Read the model definition and answer for the solid it produces. Units are mm, in the model's axes. A direction names the side the tool comes from. Coordinates: 2 decimals unless noted, no trailing zeros. Write each loop counter-clockwise with the first axis right and the second up, starting at its lowest first coordinate (ties: lowest second). Pieces come first, ordered by that corner, then holes.
Item 1: Determine the mould class of faces 1 (the face through (-4, 10, -17)), 2 (the face through (227, 15, -17)), 3 (the face through (-14, 0, -12)), 4 (the face through (232.3, 0, -11)) for opening direction X: released by +X, released by -X, zero draft, split by the parting line, or undercut.
Item 2: Straight lines are drawn through the part: probe 1 along X at (y, z) = (2, -13); probe 2 along Z at (x, y) = (94, -0.5); probe 3 along X at (y, z) = (6, -16). For each, find the intervals that lie inside material, in ascending order.
Item 3: Section A-A (y = -9) is taken. Give the vertices of the cut face in (x, z), then the cut area to 3 significant figures.
Item 4: Section D-D (x = 36) is taken. Give the vertices of the cut face in (y, z), then the cut area to 3 significant figures.
Item 5: A tool of negligible diameter and unlimited length cuts with its end or side. For faces 5 (the face through (222.3, 10, -17)), 6 (the face through (108, -5, -17)), 7 (the face through (-12, 5.63, -7)), 8 (the face through (228.3, 0, -7)), from which of +Z, -Z, +X, -X, +Y, -Y can it reach the whole face along a straight path? Write none if from no direction.
Item 6: Section B-B (z = -5.5) is taken. Give the vertices of the cut face in (x, y), then the cut area to 3 significant figures.
Item 7: Section C-C (y = 0) is taken. Give the vertices of the cut face in (x, z).
Item 8: Each of these flat-tipped pins is pushed along its axis until it touches: P1, Ø4.5, axis at x = 230, z = -7.5, coming from the -Y side; P2, Ø4.5, axis at x = 99.5, z = -17, coming from the -Y side; P3, Ø2, axis at x = 229.5, z = -10.5, coming from the +Y side. Where does it stop, or does it pass through?
from build123d import *

# Parameters (mm, degrees)
EXTRUDE_START   = -15
SKETCH_1_W      = 246.3
SKETCH_1_H      = 10
EXTRUDE_1_DEPTH = 4
SKETCH_2_W      = 10
SKETCH_2_H      = 30
EXTRUDE_2_DEPTH = 4
EXTRUDE_3_DEPTH = 4
EXTRUDE_START_2 = -4
EXTRUDE_4_DEPTH = 4


with BuildPart() as part:
    # 草图1 → 凸台-拉伸1 (new body)
    with BuildSketch(Plane.XY.offset(EXTRUDE_START)):
        with Locations((109.15, 0)):
            Rectangle(SKETCH_1_W, SKETCH_1_H)
    extrude(amount=-EXTRUDE_1_DEPTH)

    # 草图2 → 凸台-拉伸2 (add)
    with BuildSketch(Plane(origin=(0, 0, -19), x_dir=(-1, 0, 0), z_dir=(0, 0, -1))):
        with Locations((9, 0)):
            Rectangle(SKETCH_2_W, SKETCH_2_H)
        with Locations((-227.3, 0)):
            Rectangle(SKETCH_2_W, SKETCH_2_H)
    extrude(amount=-EXTRUDE_2_DEPTH)

    # 草图4 → 凸台-拉伸3 (add)
    with BuildSketch(Plane(origin=(232.3, 0, 0), x_dir=(0, 0, -1), z_dir=(1, 0, 0))):
        with BuildLine():
            Line((0, -2.63), (0, -5.63))
            Line((0, -5.63), (15, -5.63))
            Line((15, -5.63), (15, 5.63))
            Line((15, 5.63), (0, 5.63))
            Line((0, 5.63), (0, 2.63))
            ThreePointArc((0, 2.63), (2.63, 0), (0, -2.63))
        make_face()
    extrude(amount=-EXTRUDE_3_DEPTH)

    # 草图5 → 凸台-拉伸4 (add)
    with BuildSketch(Plane.ZY.offset(14).offset(EXTRUDE_START_2)):
        with BuildLine():
            Line((0, 2.63), (0, 5.63))
            Line((0, 5.63), (-15, 5.63))
            Line((-15, 5.63), (-15, -5.63))
            Line((-15, -5.63), (0, -5.63))
            Line((0, -5.63), (0, -2.63))
            ThreePointArc((0, -2.63), (-2.63, 0), (0, 2.63))
        make_face()
    extrude(amount=EXTRUDE_4_DEPTH)


solid = part.part
Established:
1. face 1: undercut
1. face 2: zero draft
1. face 3: released by -X
1. face 4: released by +X
2. probe 1: x = -14 to -10, 228.3 to 232.3
2. probe 2: z = -19 to -15
2. probe 3: x = -14 to -4, 222.3 to 232.3
3. outline: (-14, -19) - (-4, -19) - (-4, -15) - (-14, -15) - close; (222.3, -19) - (232.3, -19) - (232.3, -15) - (222.3, -15) - close
3. area: 80.0 mm2
4. outline: (-5, -19) - (5, -19) - (5, -15) - (-5, -15) - close
4. area: 40.0 mm2
5. face 5: +Z, -Z, +Y
5. face 6: +Z, -Z, -Y
5. face 7: +Z, +X, -X, +Y
5. face 8: +Z, +Y, -Y
6. outline: (-14, -5.63) - (-10, -5.63) - (-10, 5.63) - (-14, 5.63) - close; (228.3, -5.63) - (232.3, -5.63) - (232.3, 5.63) - (228.3, 5.63) - close
6. area: 90.1 mm2
7. outline: (-14, -19) - (232.3, -19) - (232.3, -2.63) - (228.3, -2.63) - (228.3, -15) - (-10, -15) - (-10, -2.63) - (-14, -2.63) - close
8. P1: stops at y = -5.63
8. P2: stops at y = -5
8. P3: stops at y = 5.63
